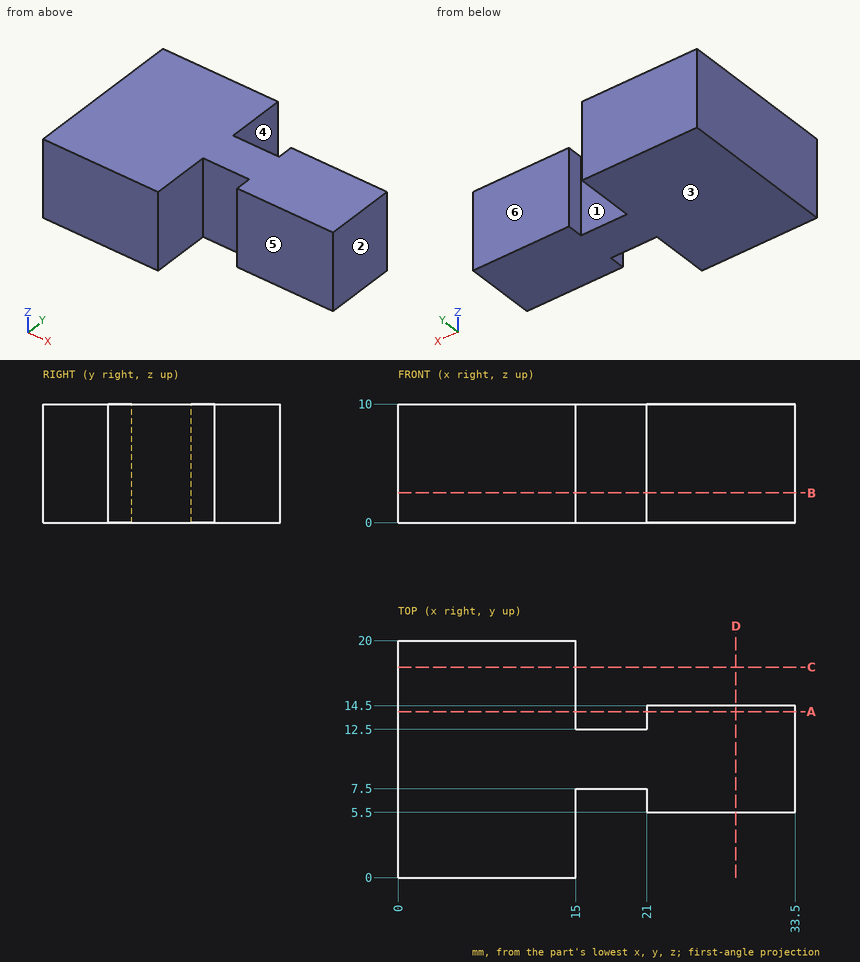
Study the drawing (mm; zero at the part's minimum x, y, z) and answer. A direction names the side the tool comes from. Round coordinates to 2 decimals unless told otherwise and drop trailing zeros. Write each loop counter-clockwise with the first axis right and the second up, starting at its lowest first coordinate (ties: lowest second). Pieces come first, ordered by that corner, then holes.
1) Straight lines are drawn through the part: line 1 (X direction, y = 6.75, z = 4.75); line 2 (X direction, y = 16.5, z = 3); line 3 (Y direction, x = 30, z = 4.5). For each, find the intervals that lie inside material, in ascending order.
2) The mould has two halves that part along X. Classify the marked faces 1, 2 and 3: pulls with the +X half, pulls with the -X half, needs draft (parallel to the pull), parting line crosses it, or undercut.
3) A cutting plane is placed at C-C (y = 17.75). Give the vertices of the cut face in (x, z).
4) A cutting plane is placed at D-D (x = 28.5). Give the vertices of the cut face in (y, z).
5) A cutting plane is placed at B-B (z = 2.5). Give the vertices of the cut face in (x, y), plus the area to 4 significant figures.
6) A cutting plane is placed at A-A (y = 14). Give the vertices of the cut face in (x, z).
7) A tool of negligible diameter and unlimited length cuts with its end or side. For the marked faces 4, 5 and 6, from which of +Z, -Z, +X, -X, +Y, -Y can it reach the whole face along a straight path? Write none if from no direction.
8) Given pin 1 Ø8 at (x, y) = (25.5, 5.5) entering from -Z; pin 2 Ø3 at (x, z) = (29.5, 3.5) entering from -Y; pin 3 Ø3 at (x, z) = (27.5, 6) entering from +Y; pin 4 Ø1.8 at (x, z) = (17, 6.5) entering from +Y, each flat-ended and moving along its own axis, determine where each tip first touches the part or whether it passes through.
Completed:
1. line 1: x = 0 to 15, 21 to 33.5
1. line 2: x = 0 to 15
1. line 3: y = 5.5 to 14.5
2. face 1: undercut
2. face 2: pulls with the +X half
2. face 3: needs draft
3. outline: (0, 0) - (15, 0) - (15, 10) - (0, 10) - close
4. outline: (5.5, 0) - (14.5, 0) - (14.5, 10) - (5.5, 10) - close
5. outline: (0, 0) - (15, 0) - (15, 7.5) - (21, 7.5) - (21, 5.5) - (33.5, 5.5) - (33.5, 14.5) - (21, 14.5) - (21, 12.5) - (15, 12.5) - (15, 20) - (0, 20) - close
5. area: 442.5 mm2
6. outline: (0, 0) - (15, 0) - (15, 10) - (0, 10) - close; (21, 0) - (33.5, 0) - (33.5, 10) - (21, 10) - close
7. face 4: +Z, -Z, +Y
7. face 5: +Z, -Z, +X, -Y
7. face 6: +Z, -Z, +X, +Y
8. pin 1: stops at z = 0
8. pin 2: stops at y = 5.5
8. pin 3: stops at y = 14.5
8. pin 4: stops at y = 12.5
